from build123d import *

# Parameters (mm, degrees)
F0_R     = 5
F1_DEPTH = 10
F2_R     = 3
F3_DEPTH = 35
F4_W     = 16
F4_H     = 14.067116
F5_DEPTH = 8


with BuildPart() as f1:
    # F0 (on Right) → F1 (new body)
    with BuildSketch(Plane.YZ):
        Circle(F0_R)
    extrude(amount=F1_DEPTH)

    # F2 (on face) → F3 (join)
    with BuildSketch(Plane.YZ.offset(10)):
        Circle(F2_R)
    extrude(amount=F3_DEPTH)

    # F4 (on face) → F5 (join)
    with BuildSketch(Plane(origin=(0, 0, 0), x_dir=(0, -1, 0), z_dir=(-1, 0, 0))):
        with Locations((0, -0.167443)):
            Rectangle(F4_W, F4_H)
    extrude(amount=F5_DEPTH)


solid = f1.part
Build history of the part. All positions in model axes, mm. A direction names the side the tool comes from. Coordinates: 2 decimals unless noted, no trailing zeros. Order: outer loops, then holes, each group sorted by start corner. A loop starts at its lowest first (then second) coordinate and runs counter-clockwise, first axis right, second up. Notation, with made-up numbers: (-14, -14.5) - (25, -14.5) arc R27 ccw to (25, 14.5) - close; hole circle Ø5 at (64.25, 35). An arc over 180 degrees is marked (long way). Put each result on its own line as item: value.
1. Probe line 1 along X through (y, z) = (2.75, 2); line 2 along X through (y, z) = (6.5, -1); line 3 along Z through (x, y) = (43, 0). List the from-to ranges inside material, lowest first. Write a range as [from, to].
Answer sheet:
line 1: x = [-8, 10]
line 2: x = [-8, 0]
line 3: z = [-3, 3]
2. Drop flat-ended pins along their axis: P1, Ø4, axis at x = 20, y = 4, coming from the -Z side; P2, Ø2, axis at x = 1.5, z = -1, coming from the +Y side; P3, Ø6, axis at x = 19, z = 4.5, coming from the +Y side. Give the stop position or say it passes through.
Answer sheet:
P1: stops at z = -2.24
P2: stops at y = 5
P3: stops at y = 2.6
3. Saw through at B-B (z = -4). Write the cut outline in (x, y).
Answer sheet:
outline: (-8, -8) - (0, -8) - (0, -3) - (10, -3) - (10, 3) - (0, 3) - (0, 8) - (-8, 8) - close
4. Saw through at C-C (x = 3). Write the cut outline in (y, z), and give its area (3 significant figures).
Answer sheet:
outline: circle Ø10 at (0, 0)
area: 78.5 mm^2
5. Saw through at D-D (z = 0). Write the cut outline in (x, y).
Answer sheet:
outline: (-8, -8) - (0, -8) - (0, -5) - (10, -5) - (10, -3) - (45, -3) - (45, 3) - (10, 3) - (10, 5) - (0, 5) - (0, 8) - (-8, 8) - close
6. Tool access for faces 1 (the face through (-8, 0, 0)), 2 (the face through (10, -0.1, -3.3)): list every direction of +Z, -Z, +X, -X, +Y, -Y with a clear straight run to the whole face (end or side of a thin tool).
Answer sheet:
face 1: +Z, -Z, -X, +Y, -Y
face 2: +X
7. Saw through at A-A (y = 0). Write the cut outline in (x, z).
Answer sheet:
outline: (-8, -7.2) - (0, -7.2) - (0, -5) - (10, -5) - (10, -3) - (45, -3) - (45, 3) - (10, 3) - (10, 5) - (0, 5) - (0, 6.87) - (-8, 6.87) - close
